```python
from build123d import *

# Parameters (mm, degrees)
F1_DEPTH = 25.4


with BuildPart() as f1:
    # F0 (on Top) → F1 (new body)
    with BuildSketch(Plane.XY):
        Polygon((76.2, -12.7), (76.2, 12.7), (-76.2, 12.7), (-76.2, -12.7), (-57.15, -12.7), (-38.1, -12.7), (-19.05, -12.7), (0, -12.7), (19.05, -12.7), (38.1, -12.7), (57.15, -12.7), align=None)
        Polygon((66.675, -20.32), (76.2, -12.7), (57.15, -12.7), align=None)
        Polygon((-57.15, -12.7), (-76.2, -12.7), (-66.675, -20.32), align=None)
        Polygon((47.625, -20.32), (57.15, -12.7), (38.1, -12.7), align=None)
        Polygon((-38.1, -12.7), (-57.15, -12.7), (-47.625, -20.32), align=None)
        Polygon((28.575, -20.32), (38.1, -12.7), (19.05, -12.7), align=None)
        Polygon((-19.05, -12.7), (-38.1, -12.7), (-28.575, -20.32), align=None)
        Polygon((9.525, -20.32), (19.05, -12.7), (0, -12.7), align=None)
        Polygon((0, -12.7), (-19.05, -12.7), (-9.525, -20.32), align=None)
    extrude(amount=F1_DEPTH)


solid = f1.part
```
Verification items for the finished model (mm, model axes). A direction names the side the tool comes from. Coordinates: 2 decimals unless noted, no trailing zeros. Write each loop counter-clockwise with the first axis right and the second up, starting at its lowest first coordinate (ties: lowest second). Pieces come first, ordered by that corner, then holes. Notation, with made-up numbers: M 33,67.25 L 81,67.25 A12 ccw 81,71.25 Z; hole C 72,31 d4. An arc over 180 degrees is marked long. Answer as a JSON object with one key per item and string values. Group by question number.
(1) Cross-section at D-D, the plane x = -50. Record the cut outline in (y, z).
(2) Gauge pin test, flat ends, axial feed: pin 1 (3 mm diameter, centred on x = -18.5, z = 10.5, fed in from -Y); pin 2 (5 mm diameter, centred on x = 21.5, z = 3, fed in from -Y); pin 3 (1.5 mm diameter, centred on x = -28.5, y = -16, fed in from -Z); pin 4 (1.5 mm diameter, centred on x = 18.5, z = 5, fed in from -Y). Record the tip position at first contact, or that the pin passes through.
(3) Cross-section at A-A, the plane z = 19.75. Record the cut outline in (x, y) (3 decimals), and give its area (3 significant figures).
(4) Cross-section at C-C, the plane x = -32. Record the cut outline in (y, z).
(5) Material ranges on line 1 (Y direction, x = 31, z = 9.5); line 2 (Y direction, x = 22.5, z = 15.5), recorded low to high.
(6) Cross-section at B-B, the plane y = -15. State how many separate pieces and enclosed holes the cut face has, and give its area (3 significant figures).
(7) Release check for a two-part mould opening along X. For faces 1 (the face through (-52.45, -16.46, 12.52)), 2 (the face through (-1, -4, 0)), 3 (the face through (42.8, -16.46, 12.52)), 4 (the face through (76.2, 0, 13)) record: +X half, -X half, draft (parallel to the pull), parting line (faces both ways), or undercut.
(8) Tool access check on faces 5 (the face through (52.321, -16.563, 12.522)), 6 (the face through (-76.2, 0, 13)). Record the directions out of +Z, -Z, +X, -X, +Y, -Y that give a thin tool (end or side, any length) a straight path to the whole face; none if there is none.
Reply:
{
 "1": {"outline": "M -18.42,0 L 12.7,0 L 12.7,25.4 L -18.42,25.4 Z"},
 "2": {"pin 1": "y = -14.34", "pin 2": "y = -16.66", "pin 3": "z = 0", "pin 4": "y = -13.74"},
 "3": {"outline": "M -76.2,-12.7 L -66.675,-20.32 L -57.15,-12.7 L -47.625,-20.32 L -38.1,-12.7 L -28.575,-20.32 L -19.05,-12.7 L -9.525,-20.32 L 0,-12.7 L 9.525,-20.32 L 19.05,-12.7 L 28.575,-20.32 L 38.1,-12.7 L 47.625,-20.32 L 57.15,-12.7 L 66.675,-20.32 L 76.2,-12.7 L 76.2,12.7 L -76.2,12.7 Z", "area": "4,450 mm²"},
 "4": {"outline": "M -17.58,0 L 12.7,0 L 12.7,25.4 L -17.58,25.4 Z"},
 "5": {"line 1": "-18.38 to 12.7", "line 2": "-15.46 to 12.7"},
 "6": {"separate pieces": "8", "enclosed holes": "0", "area": "2,700 mm²"},
 "7": {"face 1": "undercut", "face 2": "draft", "face 3": "undercut", "face 4": "+X half"},
 "8": {"face 5": "+Z, -Z, -Y", "face 6": "+Z, -Z, -X, +Y, -Y"}
}
